Source: three-view drawing plus pictorial views. Frame: mm from the lowest corner of the part. Give positions to 0.01 mm unless a question says otherwise; leave off trailing zeros. Order: outer loops, then holes, each group sorted by start corner. A loop starts at its lowest first (then second) coordinate and runs counter-clockwise, first axis right, second up.
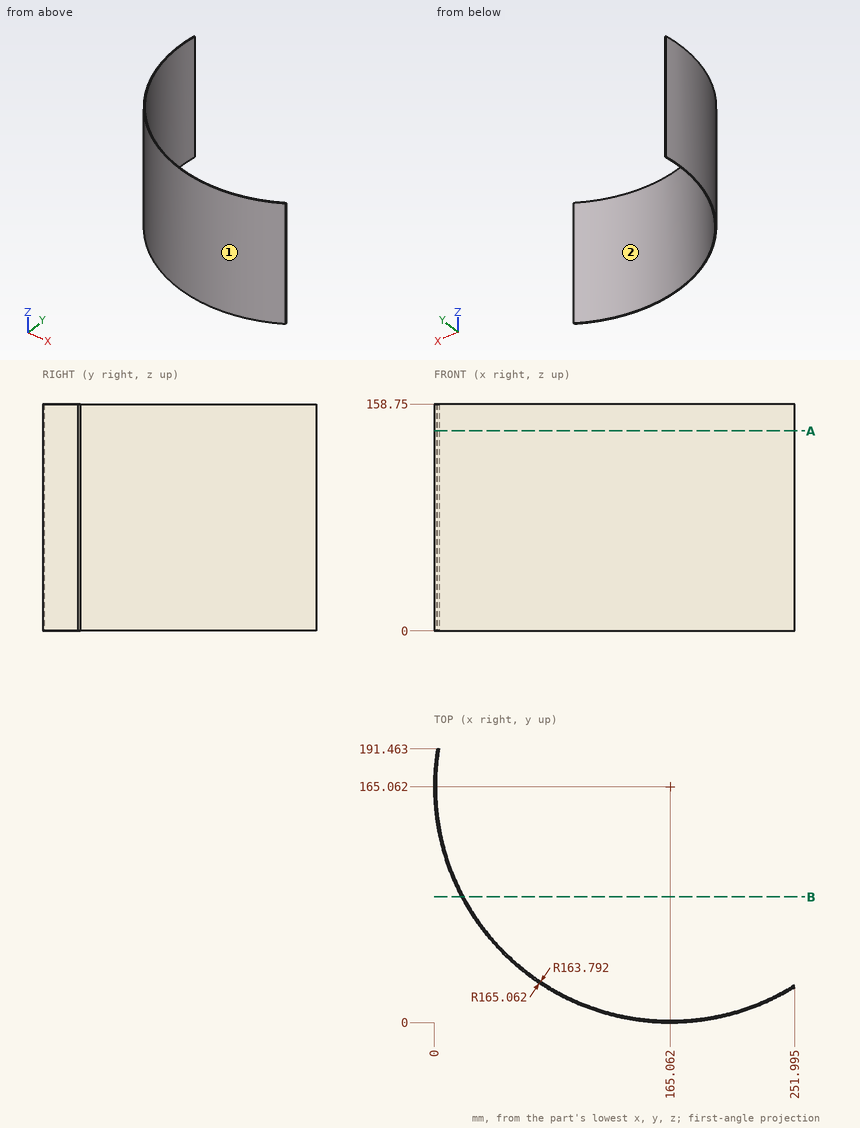
1) Section query B-B on y = 88. Output: boundary loops of the cut face in (x, z).
Checks:
outline: (19.09, 0) - (20.53, 0) - (20.53, 158.75) - (19.09, 158.75) - close
2) Section query A-A on z = 140. Output: boundary loops of the cut face in (x, y) (1 decimal).
Checks:
outline: (2.1, 191.5) arc R165.1 ccw to (252, 24.7) - (252, 26.2) arc R163.8 cw to (3.4, 191.5) - close
3) First-contact query: pin 1 Ø6 at (x, z) = (149.5, 110.5) entering from +Y (1 decimal); pin 2 Ø10 at (y, z) = (40.5, 107) entering from -X; pin 3 Ø1 at (y, z) = (65.5, 134.5) entering from -X. Flat tips, straight axial feed; report the tip coordinate or a pass-through.
Checks:
pin 1: stops at y = 2.3
pin 2: stops at x = 51.26
pin 3: stops at x = 33.03
4) Ray query, L1, parallel to X at y = 167, z = 100; L2, parallel to X at y = 33, z = 30.5 (1 decimal); L3, parallel to Y at x = 121, z = 149.5. Return the intervals inside material, ascending.
Checks:
L1: x = 0.01 to 1.28
L2: x = 66 to 68.2
L3: y = 5.99 to 7.31
5) Pull-direction query (X, two-part tool) for the marked faces 1 and 2; classes: +X half, -X half, draft (parallel to the pull), parting line (faces both ways), or undercut.
Checks:
face 1: parting line
face 2: undercut
